from build123d import *

# Parameters (mm, degrees)
SKETCH1_R           = 47.5
BOSS_EXTRUDE1_DEPTH = 30
BOSS_EXTRUDE1_DRAFT = 5
SKETCH1_3_R         = 50.5
BOSS_EXTRUDE2_DEPTH = 3
SKETCH2_R           = 50.124659906
BOSS_EXTRUDE3_DEPTH = 20


with BuildPart() as part:
    # Sketch1 → Boss-Extrude1 (with draft: the straight prism first)
    with BuildSketch(Plane.XY):
        Circle(SKETCH1_R)
    extrude(amount=-BOSS_EXTRUDE1_DEPTH)
    # Boss-Extrude1: the draft: its side faces are tilted about the plane it starts from
    boss_extrude1_sides = [part.faces().sort_by_distance(p)[0] for p in [
        (-47.5, 0, -15),
    ]]
    draft(boss_extrude1_sides, Plane.XY, BOSS_EXTRUDE1_DRAFT)

    # Sketch1<3> → Boss-Extrude2 (add)
    with BuildSketch(Plane.XY):
        Circle(SKETCH1_3_R)
    extrude(amount=-BOSS_EXTRUDE2_DEPTH)

    # Sketch2 → Boss-Extrude3 (add)
    with BuildSketch(Plane(origin=(0, 0, -30), x_dir=(-1, 0, 0), z_dir=(0, 0, -1))):
        Circle(SKETCH2_R)
    extrude(amount=BOSS_EXTRUDE3_DEPTH)


solid = part.part
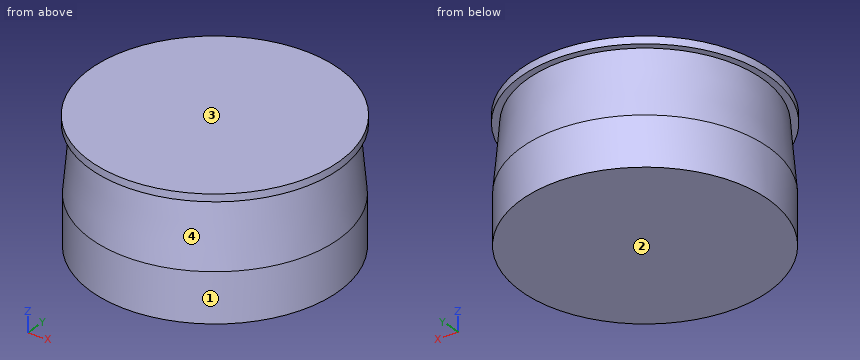
Verification items for the finished model (mm, model axes). Face numbers are marked on the shaded views. Round coordinates to 2 decimals unless told otherwise and drop trailing zeros. Write each loop counter-clockwise with the first axis right and the second up, starting at its lowest first coordinate (ties: lowest second). Pieces come first, ordered by that corner, then holes.
(1) Section check D-D (z = -12.5). Enter the section's corners in (x, y), plus the area to 3 significant figures.
Returned:
outline: circle Ø97.19 at (0, 0)
area: 7,420 mm2
(2) Material ranges on line 1 (X direction, y = 1, z = -21.5); line 2 (Y direction, x = -2.5, z = -46); line 3 (Y direction, x = -42, z = -30), recorded low to high.
Returned:
line 1: x = -49.37 to 49.37
line 2: y = -50.06 to 50.06
line 3: y = -27.36 to 27.36
(3) Depth check by flat-ended pin: pin 1 Ø3 at (y, z) = (-34.5, -24.5) entering from -X; pin 2 Ø10 at (y, z) = (-29.5, -14) entering from -X; pin 3 Ø1.5 at (x, z) = (36, -7) entering from +Y. Enter the tip coordinate at first touch or a pass-through.
Returned:
pin 1: stops at x = -37.1
pin 2: stops at x = -42.16
pin 3: stops at y = 32.75
(4) Section check A-A (z = -42). Enter the section's corners in (x, y).
Returned:
outline: circle Ø100.25 at (0, 0)
(5) Mould release check, pull along Z, two halves, no side actions. Record for the marked faces 1, 2, 3 and 4: pulls with the +Z half, pulls with the -Z half, needs draft (parallel to the pull), parting line crosses it, or undercut.
Returned:
face 1: needs draft
face 2: pulls with the -Z half
face 3: pulls with the +Z half
face 4: undercut
(6) Section check B-B (x = 0). Enter the section's corners in (y, z), plus the area to 3 significant figures.
Returned:
outline: (-50.5, -3) - (-47.76, -3) - (-50.12, -30) - (-50.12, -50) - (50.12, -50) - (50.12, -30) - (47.76, -3) - (50.5, -3) - (50.5, 0) - (-50.5, 0) - close
area: 4,950 mm2
